from build123d import *

# Parameters (mm, degrees)
SKETCH1_W            = 66
SKETCH1_H            = 36
BOSS_EXTRUDE1_DEPTH  = 1.6
M3_CLEARANCE_HOLE1_D = 3.2
MIRROR2_COPY_1_D     = 3.2


with BuildPart() as part:
    # Sketch1 → Boss-Extrude1 (new body)
    with BuildSketch(Plane(origin=(0, 0, 0), x_dir=(1, 0, 0), z_dir=(0, 1, 0))):
        Rectangle(SKETCH1_W, SKETCH1_H)
    extrude(amount=BOSS_EXTRUDE1_DEPTH)

    # M3 Clearance Hole1 (through all)
    with Locations(Plane(origin=(0, 1.6, 0), x_dir=(1, 0, 0), z_dir=(0, 1, 0))):
        with Locations((-30.5, 15.5)):
            m3_clearance_hole1 = Hole(M3_CLEARANCE_HOLE1_D / 2)

    # Mirror1: M3 Clearance Hole1 across plane
    add(m3_clearance_hole1.mirror(Plane(origin=(0, 0, 0), x_dir=(0, 0, 1), z_dir=(1, 0, 0))), mode=Mode.SUBTRACT)

    # Mirror2: M3 Clearance Hole1 across plane
    add(m3_clearance_hole1.mirror(Plane.XY), mode=Mode.SUBTRACT)

    # Mirror2 copy 1 (through all)
    with Locations(Plane(origin=(0, 1.6, 0), x_dir=(-1, 0, 0), z_dir=(0, 1, 0))):
        with Locations((-30.5, 15.5)):
            Hole(MIRROR2_COPY_1_D / 2)


solid = part.part
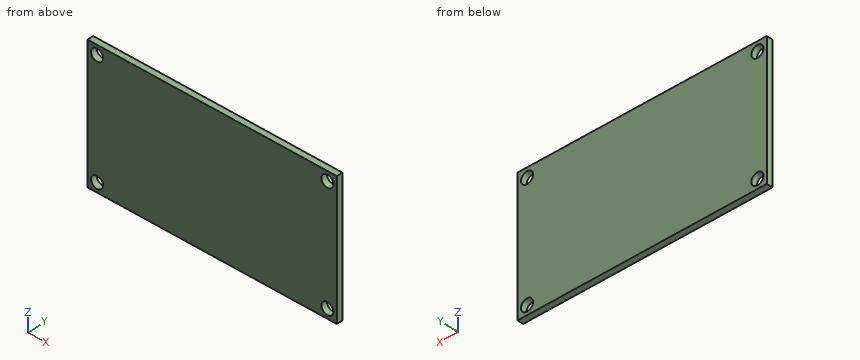
The listing builds one solid part. Answer for the finished solid, in the listing's coordinates (mm). Round coordinates to 2 decimals unless told otherwise and drop trailing zeros. Loops run counter-clockwise (first coordinate to the right, second up) from the corner with the lowest first, then second, coordinate; pieces in that order, holes last. Notation, with made-up numbers: M -34,24 L 21,24 A23 cw 21,53 Z; hole C 8,18 d1. An arc over 180 degrees is marked long. Return JSON: item names as keys, results as strings.
Q1. This flat-tipped pin is pushed along its axis until it touches: pin 1 Ø3 at (x, z) = (30.5, 15.5) entering from +Y. Where does it stop, or does it pass through?
Results list:
{"pin 1": "passes through"}
Q2. Find section B-B, the plane x = -30.5. Determine the outline of the cut face in (y, z).
Results list:
{"outline": "M 0,-18 L 1.6,-18 L 1.6,-17.1 L 0,-17.1 Z; M 0,-13.9 L 1.6,-13.9 L 1.6,13.9 L 0,13.9 Z; M 0,17.1 L 1.6,17.1 L 1.6,18 L 0,18 Z"}
Q3. Find the intervals of material crossed by line 1 along Z through (x, y) = (30.5, 0.95); line 2 along X through (y, z) = (1, -16), in increasing order. Write a range as from..to.
Results list:
{"line 1": "z = -18..-17.1, -13.9..13.9, 17.1..18", "line 2": "x = -33..-32.02, -28.98..28.98, 32.02..33"}
Q4. Find section A-A, the plane z = 15.5. Determine the outline of the cut face in (x, y), plus the area to 3 significant figures.
Results list:
{"outline": "M -33,0 L -32.1,0 L -32.1,1.6 L -33,1.6 Z; M -28.9,0 L 28.9,0 L 28.9,1.6 L -28.9,1.6 Z; M 32.1,0 L 33,0 L 33,1.6 L 32.1,1.6 Z", "area": "95.4 mm2"}
